The figure shows three views and two pictorial views of one solid part (mm, origin at its lowest corner). Answer the questions. Round coordinates to 2 decimals unless told otherwise and drop trailing zeros. Write each loop counter-clockwise with the first axis right and the second up, starting at its lowest first coordinate (ties: lowest second). Pieces come first, ordered by that corner, then holes. Notation, with made-up numbers: M 68,25 L 113,25 A19 ccw 113,56 Z; hole C 16,80.5 d7. An arc over 180 degrees is marked long. Answer in a Markdown table with one row per item.
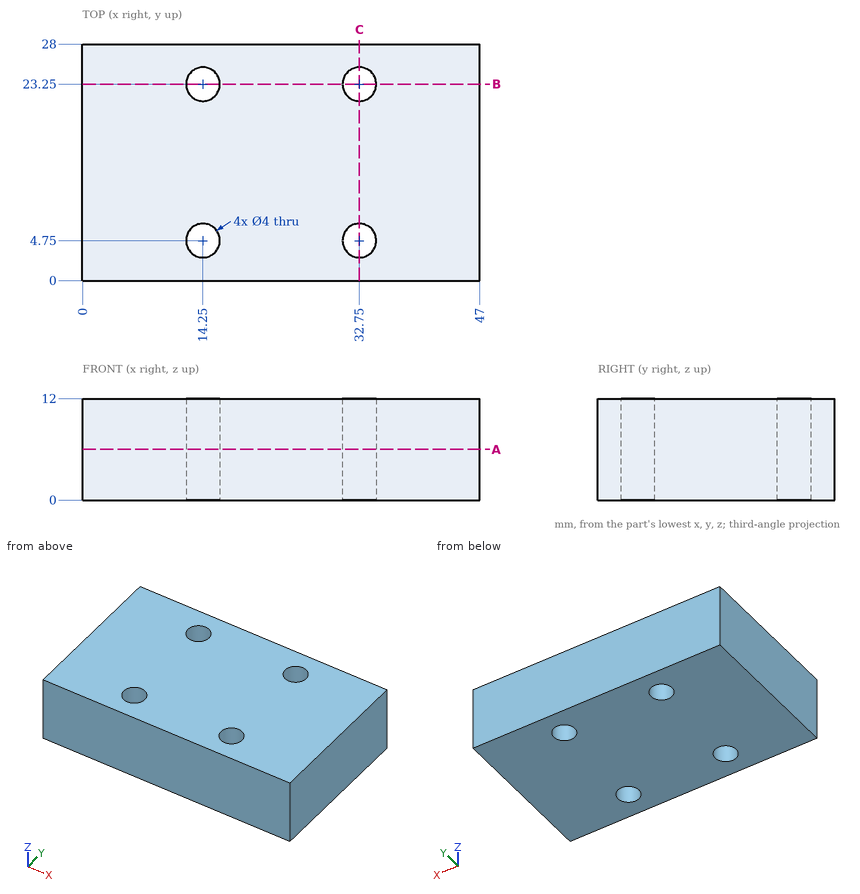
1. The part is cut by section B-B (y = 23.25). Determine the outline of the cut face in (x, z).
Calculated:
| item | result |
|---|---|
| outline | M 0,0 L 12.25,0 L 12.25,12 L 0,12 Z; M 16.25,0 L 30.75,0 L 30.75,12 L 16.25,12 Z; M 34.75,0 L 47,0 L 47,12 L 34.75,12 Z |
2. The part is cut by section C-C (x = 32.75). Determine the outline of the cut face in (y, z), plus the area to 3 significant figures.
Calculated:
| item | result |
|---|---|
| outline | M 0,0 L 2.75,0 L 2.75,12 L 0,12 Z; M 6.75,0 L 21.25,0 L 21.25,12 L 6.75,12 Z; M 25.25,0 L 28,0 L 28,12 L 25.25,12 Z |
| area | 240 mm² |
3. Consider line 1 along Y through (x, z) = (32.75, 8.5); line 2 along X through (y, z) = (22.75, 9); line 3 along X through (y, z) = (22, 5). Determine where each line is inside the solid, lowest interval first. Write a range as from..to.
Calculated:
| item | result |
|---|---|
| line 1 | y = 0..2.75, 6.75..21.25, 25.25..28 |
| line 2 | x = 0..12.31, 16.19..30.81, 34.69..47 |
| line 3 | x = 0..12.69, 15.81..31.19, 34.31..47 |
4. The part is cut by section A-A (z = 6). Determine the outline of the cut face in (x, y).
Calculated:
| item | result |
|---|---|
| outline | M 0,0 L 47,0 L 47,28 L 0,28 Z; hole C 14.25,4.75 d4; hole C 14.25,23.25 d4; hole C 32.75,4.75 d4; hole C 32.75,23.25 d4 |
